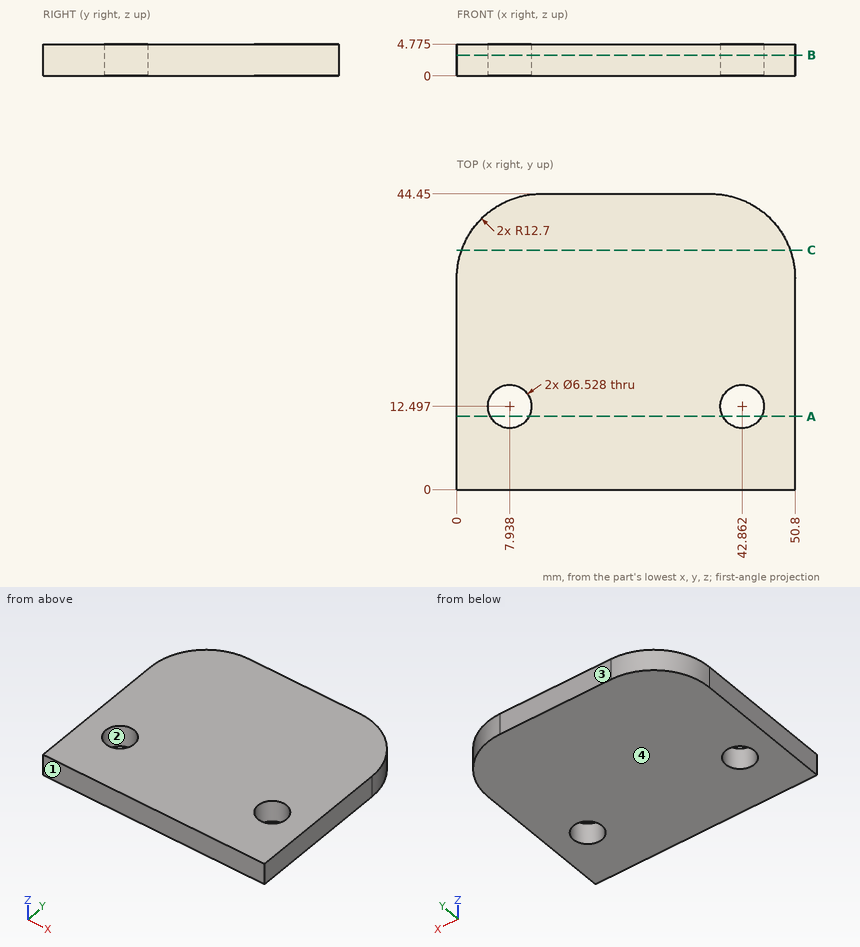
The drawing under review shows one solid part. Ordinate dimensions are in mm from its lowest x, y, z. Round coordinates to 2 decimals unless told otherwise and drop trailing zeros. Order: outer loops, then holes, each group sorted by start corner. A loop starts at its lowest first (then second) coordinate and runs counter-clockwise, first axis right, second up. Notation, with made-up numbers: (-35, 24) -> (-19, 24) arc R27 cw to (-19, 47) -> close; hole circle Ø4 at (-25.75, -31). An arc over 180 degrees is marked (long way). Use a Markdown table: item, result.
Item 1: For pin 1 (5 mm diameter, centred on x = 42.86, y = 12.5, fed in from -Z), flat-tipped, find the tip position at first contact; note if it passes through.
Resolved:
| item | result |
|---|---|
| pin 1 | passes through |
Item 2: Take a section at C-C (y = 36). State the section outline as (x, z) points (1 decimal).
Resolved:
| item | result |
|---|---|
| outline | (0.7, 0) -> (50.1, 0) -> (50.1, 4.8) -> (0.7, 4.8) -> close |
Item 3: For line 1 along Y through (x, z) = (6, 2.3) (1 decimal); line 2 along X through (y, z) = (15, 4.3) (1 decimal); line 3 along Y through (x, z) = (38.5, 0.85), list the stretches that pass through material, from the lowest coordinate up. Write a range as [from, to].
Resolved:
| item | result |
|---|---|
| line 1 | y = [0, 9.9], [15.1, 42.5] |
| line 2 | x = [0, 5.8], [10, 40.8], [45, 50.8] |
| line 3 | y = [0, 44.44] |
Item 4: Draft analysis for pull direction Y (two halves, no side actions). For the marked faces 1, 2, 3 and 4, state which applies: +Y half, -Y half, draft (parallel to the pull), parting line (faces both ways), or undercut.
Resolved:
| item | result |
|---|---|
| face 1 | -Y half |
| face 2 | undercut |
| face 3 | +Y half |
| face 4 | draft |
Item 5: Take a section at A-A (y = 11). State the section outline as (x, z) points (1 decimal).
Resolved:
| item | result |
|---|---|
| outline | (0, 0) -> (5, 0) -> (5, 4.8) -> (0, 4.8) -> close; (10.8, 0) -> (40, 0) -> (40, 4.8) -> (10.8, 4.8) -> close; (45.8, 0) -> (50.8, 0) -> (50.8, 4.8) -> (45.8, 4.8) -> close |
Item 6: Take a section at B-B (z = 3.1). State the section outline as (x, y) points, plus the area to 3 significant figures.
Resolved:
| item | result |
|---|---|
| outline | (0, 0) -> (50.8, 0) -> (50.8, 31.75) arc R12.7 ccw to (38.1, 44.45) -> (12.7, 44.45) arc R12.7 ccw to (0, 31.75) -> close; hole circle Ø6.53 at (7.94, 12.5); hole circle Ø6.53 at (42.86, 12.5) |
| area | 2,120 mm² |
